Could you check a few things on this model? Use its own coordinates, in mm. Face numbers are marked on the shaded views. Coordinates: 2 decimals unless noted, no trailing zeros. Order: outer loops, then holes, each group sorted by start corner. A loop starts at its lowest first (then second) coordinate and runs counter-clockwise, first axis right, second up. Notation, with made-up numbers: (18.25, 58) - (66.25, 58) arc R19 ccw to (66.25, 88) - close; hole circle Ø5 at (27.5, 46). An arc over 180 degrees is marked (long way). Answer as a JSON object with one key per item and string values. Group by question number.
(1) Will these pins go through, and if not, where does the flat tip stop? P1, Ø4.5, axis at x = -1, z = 2, coming from the +Y side; P2, Ø1.5, axis at y = -6, z = 1, coming from the +X side; P3, Ø3, axis at y = 15, z = 4, coming from the +X side.
(2) Please list where these lines run through material, in increasing order: probe 1 along Y at (x, z) = (0, 1.4); probe 2 along Z at (x, y) = (7, 3.5); probe 3 along X at (y, z) = (20, 2).
(3) Imagine slicing it at B-B, the plane x = 0. Write out the boundary of the cut face in (y, z).
(4) Imagine slicing it at C-C, the plane z = 2.5. Give the number of separate pieces and of enclosed holes in the cut face, and give its area (3 significant figures).
(5) We'd pull the mould along X, two halves only. Please class the marked faces 1, 2 and 3: pulls with the +X half, pulls with the -X half, needs draft (parallel to the pull), parting line crosses it, or undercut.
(6) Imagine slicing it at D-D, the plane y = 15.5. Write out the boundary of the cut face in (x, z).
(7) Imagine slicing it at A-A, the plane y = 0. Write out the boundary of the cut face in (x, z).
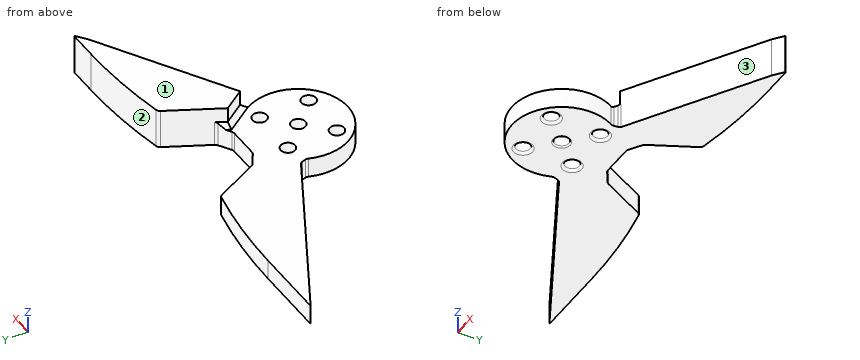
from build123d import *

# Parameters (mm, degrees)
SKETCH_1_R          = 10
EXTRUDE_1_DEPTH     = 4
EXTRUDE_3_DEPTH     = 4
SKETCH_4_R          = 1.45
CUT_EXTRUDE_1_DEPTH = 4
FILLET_5_R          = 0.5
CHAMFER_4_SIZE      = 1
EXTRUDE_START       = 4
EXTRUDE_4_DEPTH     = 4
CHAMFER_5_SIZE      = 2
CHAMFER_6_SIZE      = 1
FILLET_7_R          = 1
FILLET_8_R          = 1
FILLET_9_R          = 1
SKETCH_6_R          = 1.45
CUT_EXTRUDE_2_DEPTH = 10
FILLET_10_R         = 0.3
EXTRUDE_5_REACH     = 54.446
FILLET_11_R         = 0.1


with BuildPart() as part:
    # 草图1 → 凸台-拉伸1 (new body)
    with BuildSketch(Plane.XY):
        Circle(SKETCH_1_R)
    extrude(amount=EXTRUDE_1_DEPTH)

    # 草图3 → 凸台-拉伸3 (add)
    with BuildSketch(Plane.XY.offset(4)):
        with BuildLine():
            Line((-5.176881784364506, 11.000218871775912), (5.600807006130042, 11.000218871775912))
            Line((5.600807006130042, 11.000218871775912), (10.989651401377268, 22.000218871775843))
            ThreePointArc((10.989651401377268, 22.000218871775843), (20.91618080670068, 23.488479392998585), (30.94061356284172, 23.999999999999996))
            Line((30.94061356284172, 23.999999999999996), (0, 0))
            Line((0, 0), (-45.940613562841676, 24.00000000000002))
            Line((-45.940613562841676, 24.00000000000002), (-30.940613562841733, 23.999999999999996))
            ThreePointArc((-30.940613562841733, 23.999999999999996), (-20.916180806700666, 23.488479392998585), (-10.989651401377253, 22.000218871775836))
            Line((-10.989651401377253, 22.000218871775836), (-5.176881784364506, 11.000218871775912))
        make_face()
    extrude(amount=-EXTRUDE_3_DEPTH)

    # 草图4 → 切除-拉伸1 (cut)
    with BuildSketch(Plane(origin=(0, 0, 0), x_dir=(-1, 0, 0), z_dir=(0, 0, -1))):
        with Locations((-4.949747468305833, -4.949747468305833)):
            Circle(SKETCH_4_R)
        with Locations((-4.949747468305833, 4.949747468305833)):
            Circle(SKETCH_4_R)
        with Locations((4.949747468305833, 4.949747468305833)):
            Circle(SKETCH_4_R)
        with Locations((4.949747468305833, -4.949747468305833)):
            Circle(SKETCH_4_R)
    extrude(amount=-CUT_EXTRUDE_1_DEPTH, mode=Mode.SUBTRACT)

    # 圆角5
    fillet_5_edges = [part.edges().sort_by_distance(p)[0] for p in [
        (-3.4997474683058325, -4.949747468305833, 0),
        (-3.4997474683058325, 4.949747468305833, 0),
        (6.399747468305833, 4.949747468305833, 0),
        (6.399747468305833, -4.949747468305833, 0),
    ]]
    fillet(fillet_5_edges, radius=FILLET_5_R)

    # 倒角4
    # the kernel refuses this chamfer: 1 mm, written as the material it adds along each edge
    with BuildSketch(Plane(origin=(-8.863395681809687, 4.630358192157212, 4), x_dir=(-0.4155282844183179, -0.9095802575080274, 0), z_dir=(0, 0, -1))) as chamfer_4_piece_1:
        with BuildLine():
            Line((1.0573815899873193, -3e-17), (-CHAMFER_4_SIZE * 0.0528690794994, CHAMFER_4_SIZE * 0.998601452249))
            Line((-CHAMFER_4_SIZE * 0.0528690794994, CHAMFER_4_SIZE * 0.998601452249), (0, 0))
            ThreePointArc((0, 0), (0.5436016135552321, 0.01397436088292918), (1.0573815899873193, -3e-17))
        make_face()
    extrude(amount=4)
    with BuildSketch(Plane(origin=(7.901550123756916, 6.129070536529751, 4), x_dir=(0.5702751057051193, -0.8214537746051297, 0), z_dir=(0, 0, -1))) as chamfer_4_piece_2:
        with BuildLine():
            Line((1.0573815899873211, -5e-17), (-CHAMFER_4_SIZE * 0.0528690794994, -CHAMFER_4_SIZE * 0.998601452249))
            Line((-CHAMFER_4_SIZE * 0.0528690794994, -CHAMFER_4_SIZE * 0.998601452249), (0, 0))
            ThreePointArc((0, 0), (0.5436016135552315, -0.01397436088292837), (1.0573815899873211, -5e-17))
        make_face()
    extrude(amount=4)

    # 草图5 → 凸台-拉伸4 (add)
    with BuildSketch(Plane.XY.offset(4).offset(EXTRUDE_START)):
        with BuildLine():
            Line((10.989651401377264, 22.00021887177582), (5.600807006130042, 11.000218871775912))
            Line((5.600807006130042, 11.000218871775912), (8.691705136132603, 6.741977590182721))
            Line((8.691705136132603, 6.741977590182721), (30.94061356284172, 23.999999999999996))
            ThreePointArc((30.94061356284172, 23.999999999999996), (20.91618080670068, 23.488479392998585), (10.989651401377264, 22.00021887177582))
        make_face()
    extrude(amount=-EXTRUDE_4_DEPTH)

    # 倒角5
    chamfer_5_edges = [part.edges().sort_by_distance(p)[0] for p in [
        (-5.176881784364506, 11.000218871775912, 2),
        (5.600807006130042, 11.000218871775912, 2),
    ]]
    chamfer(chamfer_5_edges, length=CHAMFER_5_SIZE)

    # 倒角6
    chamfer_6_edges = [part.edges().sort_by_distance(p)[0] for p in [
        (7.146256071131322, 8.871098230979317, 4),
        (6.040746175985957, 11.898246447536525, 4),
    ]]
    chamfer(chamfer_6_edges, length=CHAMFER_6_SIZE)

    # 圆角7
    fillet_7_edges = [part.edges().sort_by_distance(p)[0] for p in [
        (6.480685345841874, 12.796274023297144, 2.5),
        (-3.1768817843645056, 11.00021887177591, 2),
        (3.60080700613004, 11.000218871775912, 2),
        (-6.111305934127264, 12.768509432837678, 2),
    ]]
    fillet(fillet_7_edges, radius=FILLET_7_R)

    # 圆角8
    fillet_8_edges = [part.edges().sort_by_distance(p)[0] for p in [
        (-10.989651401377252, 22.000218871775846, 2),
        (10.989651401377264, 22.000218871775836, 4),
    ]]
    fillet(fillet_8_edges, radius=FILLET_8_R)

    # 圆角9
    fillet_9_edges = [part.edges().sort_by_distance(p)[0] for p in [
        (8.504548521757462, 5.26048043823719, 2),
        (8.691705136132835, 6.741977590182982, 2.5),
        (-9.302767639872544, 3.6685847732522547, 2),
        (-9.749735249991502, 5.093394011372698, 2),
    ]]
    fillet(fillet_9_edges, radius=FILLET_9_R)

    # 草图6 → 切除-拉伸2 (cut)
    with BuildSketch(Plane(origin=(0, 0, 0), x_dir=(-1, 0, 0), z_dir=(0, 0, -1))):
        Circle(SKETCH_6_R)
    extrude(amount=-CUT_EXTRUDE_2_DEPTH, mode=Mode.SUBTRACT)

    # 圆角10
    fillet_10_edges = [part.edges().sort_by_distance(p)[0] for p in [
        (1.45, 1.8e-16, 0),
    ]]
    fillet(fillet_10_edges, radius=FILLET_10_R)

    # 凸台-拉伸5: up to this face of the body (flat: up to its plane)
    extrude_5_end = Plane(part.part.faces().sort_by_distance((-5.497293507, 11.434254101, 0))[0])
    # 草图7 → 凸台-拉伸5 (add, up to the picked face)
    with BuildSketch(Plane.XY.offset(8), mode=Mode.PRIVATE) as extrude_5_sk1:
        Polygon((30.94061356284172, 23.999999999999996), (36.94061356284172, 23.999999999999993), (34.761147405505504, 22.309432756728267), (8.691705136132603, 6.741977590182721), (28.761147405505504, 22.30943275672827), align=None)
    extrude_5_tool1 = split(extrude(extrude_5_sk1.sketch, amount=-EXTRUDE_5_REACH, mode=Mode.PRIVATE), bisect_by=extrude_5_end, keep=Keep.BOTH, mode=Mode.PRIVATE)
    add(extrude_5_tool1.solids().sort_by(Axis((25.637932, 18.197049, 8), (0, 0, -1)))[0])

    # 圆角11
    fillet_11_edges = [part.edges().sort_by_distance(p)[0] for p in [
        (36.94061356284172, 23.999999999999993, 4),
    ]]
    fillet(fillet_11_edges, radius=FILLET_11_R)


solid = part.part
Result set:
{
 "1": {"P1": "stops at y = 11.06", "P2": "stops at x = 8.51", "P3": "stops at x = 25.03"},
 "2": {"probe 1": "y = -10 to -1.45, 1.45 to 11", "probe 2": "z = 0 to 4", "probe 3": "x = -38.28 to -9.93, 10.01 to 30.89"},
 "3": {"outline": "(-10, 0) - (-1.75, 0) arc R0.3 ccw to (-1.45, 0.3) - (-1.45, 4) - (-10, 4) - close; (1.45, 0.3) arc R0.3 ccw to (1.75, 0) - (11, 0) - (11, 4) - (1.45, 4) - close"},
 "4": {"separate pieces": "1", "enclosed holes": "5", "area": "914 mm^2"},
 "5": {"face 1": "needs draft", "face 2": "undercut", "face 3": "pulls with the +X half"},
 "6": {"outline": "(-29.67, 0) - (-7.55, 0) - (-7.55, 4) - (-29.67, 4) - close; (7.81, 0) - (23.36, 0) - (23.36, 8) - (7.81, 8) - close"},
 "7": {"outline": "(-10, 0) - (-1.75, 0) arc R0.3 ccw to (-1.45, 0.3) - (-1.45, 4) - (-10, 4) - close; (1.45, 0.3) arc R0.3 ccw to (1.75, 0) - (10, 0) - (10, 4) - (1.45, 4) - close"}
}
